For this review, take the finished solid that the model builds, in its own axes (mm). Round coordinates to 2 decimals unless told otherwise and drop trailing zeros. Write each loop counter-clockwise with the first axis right and the second up, starting at its lowest first coordinate (ties: lowest second). Pieces come first, ordered by that corner, then holes. Notation, with made-up numbers: (11, 10) -> (32, 10) arc R15 cw to (32, 33) -> close; hole circle Ø9 at (-23.5, 57). An arc over 180 degrees is marked (long way). Answer as CSV lines item,"result". Start each with the question number.
Item 1: Take a section at A-A on z = -12.7. Give the boundary of the cut face in (x, y), then the cut area to 3 significant figures.
Item 2: Take a section at B-B on x = 0. Give the boundary of the cut face in (y, z) (3 decimals), then the cut area to 3 significant figures.
Item 3: Wall thickness on probe 1 along X at (y, z) = (1.5, -12.7); probe 2 along X at (y, z) = (2.5, -14): over which ranges is each line inside the solid? List them lowest first. Write a range as from..to.
Item 4: Mouldability with a two-part tool opening along X and no side actions: class faces 1 (the cylindrical face through (-0.662, 3.131, -14.295)), 2 (the flat face through (63.5, 3, 0)), 3 (the flat face through (-63.5, 3, 0)) as +X half, -X half, draft (parallel to the pull), parting line (faces both ways), or undercut.
```python
from build123d import *

# Parameters (mm, degrees)
SKETCH1_W                 = 127
SKETCH1_H                 = 44.45
BOSS_EXTRUDE1_DEPTH       = 6.35
F_8_32_TAPPED_HOLE1_D     = 3.4544
F_8_32_TAPPED_HOLE1_DEPTH = 12.446
F_8_32_TAPPED_HOLE1_TIP   = 1.037806461


with BuildPart() as part:
    # Sketch1 → Boss-Extrude1 (new body)
    with BuildSketch(Plane(origin=(0, 0, 0), x_dir=(1, 0, 0), z_dir=(0, 1, 0))):
        Rectangle(SKETCH1_W, SKETCH1_H)
    extrude(amount=BOSS_EXTRUDE1_DEPTH)

    # #8-32 Tapped Hole1
    with Locations(Plane(origin=(0, 6.35, -12.7), x_dir=(0, 0, 1), z_dir=(0, 1, 0))):
        with Locations((0, 0)):
            Hole(F_8_32_TAPPED_HOLE1_D / 2, depth=F_8_32_TAPPED_HOLE1_DEPTH)
            with Locations((0, 0, -(F_8_32_TAPPED_HOLE1_DEPTH + F_8_32_TAPPED_HOLE1_TIP / 2))):  # 118° drill point
                Cone(0, F_8_32_TAPPED_HOLE1_D / 2, F_8_32_TAPPED_HOLE1_TIP, mode=Mode.SUBTRACT)


solid = part.part
```
Output values:
1,outline,"(-63.5, 0) -> (-1.73, 0) -> (-1.73, 6.35) -> (-63.5, 6.35) -> close; (1.73, 0) -> (63.5, 0) -> (63.5, 6.35) -> (1.73, 6.35) -> close"
1,area,"785 mm^2"
2,outline,"(0, -22.225) -> (6.35, -22.225) -> (6.35, -14.427) -> (0, -14.427) -> close; (0, -10.973) -> (6.35, -10.973) -> (6.35, 22.225) -> (0, 22.225) -> close"
2,area,"260 mm^2"
3,probe 1,"x = -63.5..-1.73, 1.73..63.5"
3,probe 2,"x = -63.5..-1.14, 1.14..63.5"
4,face 1,"undercut"
4,face 2,"+X half"
4,face 3,"-X half"
